```python
from build123d import *

# Parameters (mm, degrees)
SKETCH_1_W          = 42
SKETCH_1_H          = 50
EXTRUDE_1_DEPTH     = 2
SKETCH_3_W          = 3
SKETCH_3_H          = 6
EXTRUDE_2_DEPTH     = 12
FILLET_1_R          = 5
FILLET_2_R          = 5
SKETCH_4_R          = 1
CUT_EXTRUDE_1_DEPTH = 39.013155617
SKETCH_5_R          = 2.5
EXTRUDE_3_DEPTH     = 3
SKETCH_6_W          = 9
SKETCH_6_H          = 12.266046359
CUT_EXTRUDE_2_DEPTH = 35.785054262
SKETCH_7_R          = 1.65
CUT_EXTRUDE_3_DEPTH = 36.524639337
FILLET_3_R          = 3


with BuildPart() as part:
    # 草图1 → 凸台-拉伸1 (new body)
    with BuildSketch(Plane.XY):
        Rectangle(SKETCH_1_W, SKETCH_1_H)
    extrude(amount=EXTRUDE_1_DEPTH)

    # 草图3 → 凸台-拉伸2 (add)
    with BuildSketch(Plane(origin=(0, 0, 0), x_dir=(-1, 0, 0), z_dir=(0, 0, -1))):
        with Locations((3.5, -22)):
            Rectangle(SKETCH_3_W, SKETCH_3_H)
        with Locations((3.5, 7)):
            Rectangle(SKETCH_3_W, SKETCH_3_H)
    extrude(amount=EXTRUDE_2_DEPTH)

    # 圆角1
    fillet_1_edges = [part.edges().sort_by_distance(p)[0] for p in [
        (-2, 7, 0),
    ]]
    fillet(fillet_1_edges, radius=FILLET_1_R)

    # 圆角2
    fillet_2_edges = [part.edges().sort_by_distance(p)[0] for p in [
        (-2, -22, 0),
    ]]
    fillet(fillet_2_edges, radius=FILLET_2_R)

    # 草图4 → 切除-拉伸1 (cut, through all)
    with BuildSketch(Plane.ZY.offset(5)):
        with Locations((-6.9, -20.6)):
            Circle(SKETCH_4_R)
        with Locations((-6.9, 6.3)):
            Circle(SKETCH_4_R)
    extrude(amount=-CUT_EXTRUDE_1_DEPTH, mode=Mode.SUBTRACT)

    # 草图5 → 凸台-拉伸3 (add)
    with BuildSketch(Plane(origin=(21, 0, 0), x_dir=(0, 0, -1), z_dir=(1, 0, 0))):
        with BuildLine():
            Line((0, -4.733953641), (0, -12.733953641))
            Line((0, -12.733953641), (3.333333333, -15.715377611))
            ThreePointArc((3.333333333, -15.715377611), (9.249103106, -15.067047939), (7.972848445, -9.254317307))
            Line((7.972848445, -9.254317307), (0, -4.733953641))
        make_face()
        with Locations(Location((6, -12.733953641, 0), (0, 0, 90))):
            Circle(SKETCH_5_R, mode=Mode.SUBTRACT)
    extrude(amount=-EXTRUDE_3_DEPTH)

    # 草图6 → 切除-拉伸2 (cut, through all)
    with BuildSketch(Plane(origin=(0, 0, 0), x_dir=(-1, 0, 0), z_dir=(0, 0, -1))):
        with Locations((-16.5, -18.86697682)):
            Rectangle(SKETCH_6_W, SKETCH_6_H)
        with Locations((16.5, -18.86697682)):
            Rectangle(SKETCH_6_W, SKETCH_6_H)
    extrude(amount=-CUT_EXTRUDE_2_DEPTH, mode=Mode.SUBTRACT)

    # 草图7 → 切除-拉伸3 (cut, through all)
    with BuildSketch(Plane.XY.offset(2)):
        with Locations((9.975799492, 17.266046359)):
            Circle(SKETCH_7_R)
        with Locations((-10.024200508, 17.266046359)):
            Circle(SKETCH_7_R)
    extrude(amount=-CUT_EXTRUDE_3_DEPTH, mode=Mode.SUBTRACT)

    # 圆角3
    fillet_3_edges = [part.edges().sort_by_distance(p)[0] for p in [
        (-3.5, -25, -12),
    ]]
    fillet(fillet_3_edges, radius=FILLET_3_R)


solid = part.part
```
Could you check a few things on this model? Use its own coordinates, in mm. A direction names the side the tool comes from. Give positions to 0.01 mm unless a question says otherwise; leave off trailing zeros. Order: outer loops, then holes, each group sorted by start corner. A loop starts at its lowest first (then second) coordinate and runs counter-clockwise, first axis right, second up.
Q1. We'd pull the mould along Y, two halves only. Please class faces 4 (the flat face through (-21, 6, 1)), 5 (the cylindrical face through (-3.52, -19.61, -7.03)), 6 (the flat face through (19.52, -14.2, -1.64)): +Y half, -Y half, draft (parallel to the pull), parting line (faces both ways), or undercut.
Q2. Suppose I cut it at A-A, the plane y = 6.3. Write out the boundary of the cut face in (x, z).
Q3. If I drill on line 1 along Y through (x, z) = (-2.8, -6.9); line 2 along X through (y, z) = (-14.5, -8.5); line 3 along X through (y, z) = (-20, 0.5), over which ranges is the centre line in solid material (lowest first)?
Q4. Suppose I cut it at D-D, the plane y = -20.6. Write out the boundary of the cut face in (x, z), and give its area (3 significant figures).
Q5. For faces 1 (the flat face through (-16, -12.734, 1)), 2 (the flat face through (-2, -22, -8)), 3 (the flat face through (-5, 7, -5.9)), which set-ups out of +Z, -Z, +X, -X, +Y, -Y let a thin tool reach every point of the face, with its end or its side?
Q6. I'm going to push flat-ended pins straight in: P1, Ø2, axis at x = 16, z = 1, coming from the -Y side; P2, Ø5, axis at y = -13.5, z = -6.5, coming from the -X side; P3, Ø0.6, axis at y = -20, z = 1.5, coming from the -X side; P4, Ø4, axis at y = -12.73, z = -6, coming from the -X side. Where does each tip first touch, or does it pass through?
Q7. Suppose I cut it at B-B, the plane x = -4. Write out the boundary of the cut face in (y, z).
Q8. Suppose I cut it at C-C, the plane z = -6.9. Write out the boundary of the cut face in (x, y).
Solution:
1. face 4: draft
1. face 5: undercut
1. face 6: -Y half
2. outline: (-21, 0) - (-5, 0) - (-5, -5.9) - (-2, -5.9) - (-2, -5) arc R5 cw to (3, 0) - (21, 0) - (21, 2) - (-21, 2) - close; (-5, -12) - (-2, -12) - (-2, -7.9) - (-5, -7.9) - close
3. line 1: y = -25 to -21.6, -19.6 to -19, 4 to 5.3, 7.3 to 10
3. line 2: x = 18 to 21
3. line 3: x = -12 to 12
4. outline: (-12, 0) - (-5, 0) - (-5, -5.9) - (-2, -5.9) - (-2, -5) arc R5 cw to (3, 0) - (12, 0) - (12, 2) - (-12, 2) - close; (-5, -12) - (-2, -12) - (-2, -7.9) - (-5, -7.9) - close
4. area: 83.4 mm2
5. face 1: +Z, -Z, -X, -Y
5. face 2: -Z, +X, +Y, -Y
5. face 3: -Z, -X, +Y, -Y
6. P1: stops at y = -12.73
6. P2: stops at x = 18
6. P3: stops at x = -12
6. P4: passes through
7. outline: (-25, -9) arc R3 ccw to (-22, -12) - (-19, -12) - (-19, 0) - (4, 0) - (4, -12) - (10, -12) - (10, 0) - (25, 0) - (25, 2) - (-25, 2) - close; hole circle Ø2 at (-20.6, -6.9); hole circle Ø2 at (6.3, -6.9)
8. outline: (-5, -25) - (-2, -25) - (-2, -21.6) - (-5, -21.6) - close; (-5, -19.6) - (-2, -19.6) - (-2, -19) - (-5, -19) - close; (-5, 4) - (-2, 4) - (-2, 5.3) - (-5, 5.3) - close; (-5, 7.3) - (-2, 7.3) - (-2, 10) - (-5, 10) - close; (18, -16.63) - (21, -16.63) - (21, -15.07) - (18, -15.07) - close; (18, -10.4) - (21, -10.4) - (21, -8.65) - (18, -8.65) - close
